Check sheet for the modelled part. Datum: model origin and axes. Units: mm. Face numbers are marked on the shaded views. Give positions to 0.01 mm unless a question says otherwise; leave off trailing zeros. Order: outer loops, then holes, each group sorted by start corner. A loop starts at its lowest first (then second) coordinate and runs counter-clockwise, first axis right, second up.
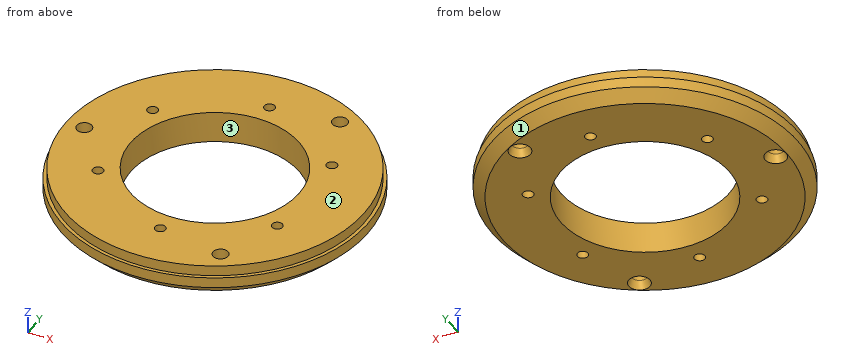
from build123d import *

# Parameters (mm, degrees)
SKETCH_R         = 50.425
PAD_DEPTH        = 7
SKETCH001_R      = 49.3
PAD001_DEPTH     = 3.5
CHAMFER_SIZE     = 3.5
SKETCH002_R      = 27.8
SKETCH002_R_2    = 2.5
SKETCH002_R_3    = 1.75
POCKET_DEPTH     = 10.501
CHAMFER001_ANGLE = 70
CHAMFER001_SIZE  = 1


with BuildPart() as part:
    # Sketch → Pad (new body)
    with BuildSketch(Plane.XY):
        Circle(SKETCH_R)
    extrude(amount=PAD_DEPTH)

    # Sketch001 (on Face3 of Pad) → Pad001 (join)
    with BuildSketch(Plane.XY.offset(7)):
        Circle(SKETCH001_R)
    extrude(amount=PAD001_DEPTH)

    # Chamfer
    chamfer_edges = [part.edges().sort_by_distance(p)[0] for p in [
        (-50.425, 0, 0),
    ]]
    chamfer(chamfer_edges, length=CHAMFER_SIZE)

    # Sketch002 (on Face6 of Chamfer) → Pocket (cut, through all)
    with BuildSketch(Plane.XY.offset(10.5)):
        Circle(SKETCH002_R)
        with Locations((-43.3, 0)):
            Circle(SKETCH002_R_2)
        with Locations((21.65, 37.4989)):
            Circle(SKETCH002_R_2)
        with Locations((21.65, -37.4989)):
            Circle(SKETCH002_R_2)
        with Locations((-29.704671, 17.15)):
            Circle(SKETCH002_R_3)
        with Locations((0, 34.3)):
            Circle(SKETCH002_R_3)
        with Locations((29.704671, 17.15)):
            Circle(SKETCH002_R_3)
        with Locations((29.704671, -17.15)):
            Circle(SKETCH002_R_3)
        with Locations((0, -34.3)):
            Circle(SKETCH002_R_3)
        with Locations((-29.704671, -17.15)):
            Circle(SKETCH002_R_3)
    extrude(amount=-POCKET_DEPTH, mode=Mode.SUBTRACT)

    # Chamfer001
    chamfer001_edges = [part.edges().sort_by_distance(p)[0] for p in [
        (19.15, -37.4989, 0),
        (-45.8, 0, 0),
        (19.15, 37.4989, 0),
    ]]
    chamfer001_side = part.faces().sort_by_distance((-46.792276, 0, 0))[0]
    chamfer(chamfer001_edges, length=CHAMFER001_SIZE, angle=CHAMFER001_ANGLE, reference=chamfer001_side)


solid = part.part
1) Section check A-A, the plane x = 0. Record the cut outline in (y, z) (3 decimals), then the cut area to 4 significant figures.
Recorded:
outline: (-50.425, 3.5) - (-46.925, 0) - (-36.05, 0) - (-36.05, 10.5) - (-49.3, 10.5) - (-49.3, 7) - (-50.425, 7) - close; (-32.55, 0) - (-27.8, 0) - (-27.8, 10.5) - (-32.55, 10.5) - close; (27.8, 0) - (32.55, 0) - (32.55, 10.5) - (27.8, 10.5) - close; (36.05, 0) - (46.925, 0) - (50.425, 3.5) - (50.425, 7) - (49.3, 7) - (49.3, 10.5) - (36.05, 10.5) - close
area: 381.5 mm2
2) Section check B-B, the plane y = 0. Record the cut outline in (x, z) (3 decimals), then the cut area to 3 significant figures.
Recorded:
outline: (-50.425, 3.5) - (-46.925, 0) - (-46.8, 0) - (-45.8, 2.747) - (-45.8, 10.5) - (-49.3, 10.5) - (-49.3, 7) - (-50.425, 7) - close; (-40.8, 2.747) - (-39.8, 0) - (-27.8, 0) - (-27.8, 10.5) - (-40.8, 10.5) - close; (27.8, 0) - (46.925, 0) - (50.425, 3.5) - (50.425, 7) - (49.3, 7) - (49.3, 10.5) - (27.8, 10.5) - close
area: 400 mm2
3) Material ranges on L1, parallel to Y at x = 0, z = 6.25 (3 decimals); L2, parallel to Y at x = -13, z = 9.5; L3, parallel to Y at x = 31, z = 3.75, recorded low to high.
Recorded:
L1: y = -50.425 to -36.05, -32.55 to -27.8, 27.8 to 32.55, 36.05 to 50.425
L2: y = -47.56 to -24.57, 24.57 to 47.56
L3: y = -39.77 to -18.33, -15.97 to 15.97, 18.33 to 39.77
4) Depth check by flat-ended pin: pin 1 Ø1.5 at (y, z) = (-31, 1.5) entering from +X; pin 2 Ø3 at (y, z) = (-15.5, 7) entering from -X; pin 3 Ø6 at (y, z) = (-10, 4) entering from +X. Enter the tip coordinate at first touch or a pass-through.
Recorded:
pin 1: stops at x = 38.35
pin 2: stops at x = -48.44
pin 3: stops at x = 49.94
5) Section check C-C, the plane y = 17.15. State how many separate pieces and enclosed holes the cut face has, then the cut area to 3 significant figures.
Recorded:
separate pieces: 4
enclosed holes: 0
area: 441 mm2
6) Draft check along Y on the marked faces 1, 2 and 3. Enter one of: +Y half, -Y half, draft (parallel to the pull), parting line (faces both ways), or undercut.
Recorded:
face 1: parting line
face 2: draft
face 3: undercut
